Read the model definition and answer for the solid it produces. Units are mm, in the model's axes. A direction names the side the tool comes from. Give positions to 0.01 mm unless a question says otherwise; leave off trailing zeros. Loops run counter-clockwise (first coordinate to the right, second up) from the corner with the lowest first, then second, coordinate; pieces in that order, holes last. Notation, with made-up numbers: (39.25, 45) - (51.25, 45) arc R15 ccw to (51.25, 74) - close; hole circle Ø5 at (5.25, -11.75). An arc over 180 degrees is marked (long way). Write item = value, one per line. Start each with the question number.
from build123d import *

# Parameters (mm, degrees)
SWEEP_THIN2_PROFILE_R   = 10
SWEEP_THIN2_PROFILE_R_2 = 7
CUT_EXTRUDE1_DEPTH      = 500.751926697
CUT_EXTRUDE1_DEPTH_BACK = 500.751926697
SKETCH22_R              = 5
SWEEP_THIN3_START       = -9.711313495
SWEEP_THIN3_OUTLINE_R   = 10
SWEEP_THIN3_OUTLINE_R_2 = 7
SWEEP_THIN3_DEPTH       = 140


with BuildPart() as part:
    # Sweep-Thin2: sweep along a path in Sketch1
    with BuildLine(Plane(origin=(0, 0, 0), x_dir=(1, 0, 0), z_dir=(0, 1, 0))) as sweep_thin2_path:
        Line((0, 0), (-73.530781703, 202.024162363))
        ThreePointArc((-73.530781703, 202.024162363), (-91.836590924, 225.880757411), (-120.515412742, 234.923155196))
        Line((-120.515412742, 234.923155196), (-435.505035831, 234.923155196))
    # Sweep-Thin2 profile (on start of the path) → Sweep-Thin2 (sweep)
    with BuildSketch(Plane(origin=(0, 0, 0), x_dir=(-0.9396926207859093, 0, 0.3420201433256662), z_dir=(-0.3420201433256662, 0, -0.9396926207859093))):
        Circle(SWEEP_THIN2_PROFILE_R)
        Circle(SWEEP_THIN2_PROFILE_R_2, mode=Mode.SUBTRACT)
    sweep(path=sweep_thin2_path.line)

    # Sketch22 → Cut-Extrude1 (cut, two sides: drawn at the far end of the back side and taken through both)
    with BuildSketch(Plane(origin=(0, 0, 0), x_dir=(1, 0, 0), z_dir=(0, 1, 0)).offset(-CUT_EXTRUDE1_DEPTH_BACK)):
        with Locations(Location((-17.101007166, 46.984631039, 0), (0, 0, 270))):
            Circle(SKETCH22_R)
    extrude(amount=CUT_EXTRUDE1_DEPTH + CUT_EXTRUDE1_DEPTH_BACK, mode=Mode.SUBTRACT)

    # Sweep-Thin3: read off the stored shape, not the designer's step
    # Sweep-Thin3 outline → Sweep-Thin3 (add)
    with BuildSketch(Plane(origin=(0, 0, 0), x_dir=(0.906307787036651, 0, 0.42261826174069705), z_dir=(0.42261826174069705, 0, -0.9063077870366512)).offset(SWEEP_THIN3_START)):
        with Locations((-276.470551871, 0)):
            Circle(SWEEP_THIN3_OUTLINE_R)
        with Locations((-276.470551871, 0)):
            Circle(SWEEP_THIN3_OUTLINE_R_2, mode=Mode.SUBTRACT)
    extrude(amount=SWEEP_THIN3_DEPTH)


solid = part.part
1. For a pull along X with two mould halves and no side action, classify faces 1 (the cylindrical face through (-200.277, -0.109, -224.924)), 2 (the flat face through (6.4, 2.36, -2.33)), 3 (the flat face through (-260.841, -2.362, -110.917)) as released by +X, released by -X, zero draft, split by the parting line, or undercut.
2. Consider line 1 along X through (y, z) = (4.25, -108); line 2 along X through (y, z) = (-6.25, -55); line 3 along Z through (x, y) = (-395.5, -0.25). Determine where each line is inside the solid, lowest interval first. Write a range as [from, to].
3. A cutting plane is placed at C-C on x = -252.5. Give the number of separate pieces and of enclosed holes in the cut face, and give its area (3 significant figures).
4. A tool of negligible diameter and unlimited length cuts with its end or side. For faces 4 (the cylindrical face through (-20.143, -7.486, -50.952)), 5 (the flat face through (-202.1, 0.5, -238)), from which of +Z, -Z, +X, -X, +Y, -Y can it reach the whole face along a straight path? Write none if from no direction.
5. Given P1, Ø1, axis at y = 3, z = -85.5, coming from the +X side; P2, Ø2, axis at x = -283.5, y = -2.5, coming from the -Z side; P3, Ø3, axis at y = -7.5, z = -36.5, coming from the -X side; P4, Ø8, axis at x = -17.1, z = -46.98, coming from the -Y side, each flat-ended and moving along its own axis, determine where each tip first touches the part or whether it passes through.
6. A cutting plane is placed at B-B on x = -395. Give the vertices of the cut face in (y, z).
Reply:
q1.face_1 = undercut
q1.face_2 = released by +X
q1.face_3 = released by -X
q2.line_1 = [-248.55, -244.7], [-48.94, -45.23], [-33.39, -29.68]
q2.line_2 = [-28.33, -23.37], [-16.66, -11.71]
q2.line_3 = [-244.92, -241.92], [-227.93, -224.93]
q3.separate_pieces = 2
q3.enclosed_holes = 1
q3.area = 384 mm^2
q4.face_4 = +Y, -Y
q4.face_5 = none
q5.P1 = -20.73
q5.P2 = -244.81
q5.P3 = -21.92
q5.P4 = through
q6.outline = circle Ø20 at (0, -234.92); hole circle Ø14 at (0, -234.92)
